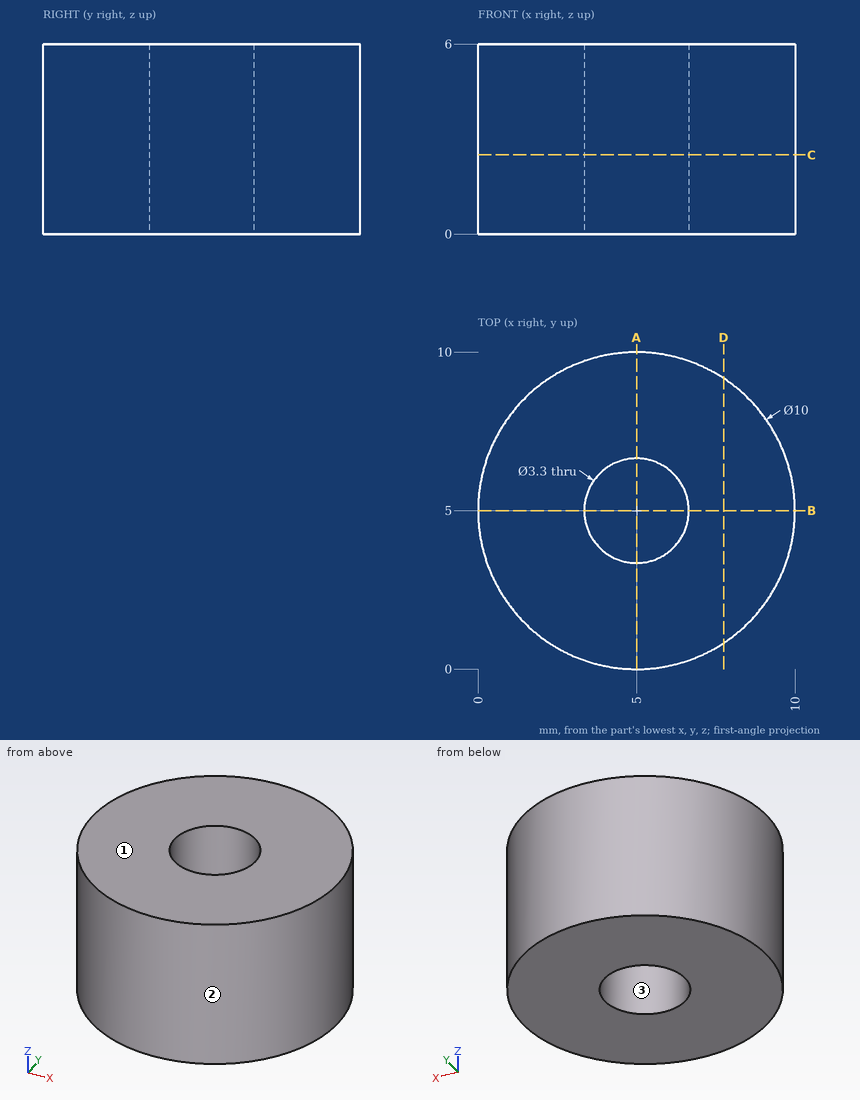
For this review, use the dimensioned drawing (mm, ordinates from the lowest corner) and the shaded views. Give positions to 0.01 mm unless a question says otherwise; leave off trailing zeros. Write each loop counter-clockwise with the first axis right and the second up, starting at its lowest first coordinate (ties: lowest second). Pieces come first, ordered by that corner, then holes.
(1) The part is to be moulded in two halves that separate along Y. For the marked faces 1, 2 and 3, say which applies: released by +Y, released by -Y, zero draft, split by the parting line, or undercut.
(2) To check wall thickness, follow L1, parallel to Y at x = 5, z = 4.25; L2, parallel to Y at x = 5.75, z = 4.55; L3, parallel to X at y = 6.25, z = 5.2. State the ranges of each line that lie inside material, in increasing order.
(3) Consider section A-A, the plane x = 5. Give the boundary of the cut face in (y, z).
(4) For P1, Ø1, axis at y = 7.5, z = 1, coming from the -X side; P2, Ø1.5, axis at x = 3, z = 4.5, coming from the +Y side; P3, Ø1.5, axis at y = 7.5, z = 4.5, coming from the +X side, all flat-tipped, find the tip position at first contact; note any pin that passes through.
(5) Consider section C-C, the plane z = 2.5. Give the boundary of the cut face in (x, y), and give its area (3 significant figures).
(6) Consider section D-D, the plane x = 7.75. Give the boundary of the cut face in (y, z).
Returned:
1. face 1: zero draft
1. face 2: split by the parting line
1. face 3: undercut
2. L1: y = 0 to 3.35, 6.65 to 10
2. L2: y = 0.06 to 3.53, 6.47 to 9.94
2. L3: x = 0.16 to 3.92, 6.08 to 9.84
3. outline: (0, 0) - (3.35, 0) - (3.35, 6) - (0, 6) - close; (6.65, 0) - (10, 0) - (10, 6) - (6.65, 6) - close
4. P1: stops at x = 0.42
4. P2: stops at y = 9.84
4. P3: stops at x = 9.68
5. outline: circle Ø10 at (5, 5); hole circle Ø3.3 at (5, 5)
5. area: 70.0 mm2
6. outline: (0.82, 0) - (9.18, 0) - (9.18, 6) - (0.82, 6) - close
